Autodesk Inventor part; units mm, degrees
ref_plane "YZ Plane" through (0, 0, 0) normal (1, 0, 0) x (0, 1, 0)
ref_plane "XZ Plane" through (0, 0, 0) normal (0, 1, 0) x (-1, 0, 0)
ref_plane "XY Plane" through (0, 0, 0) normal (0, 0, 1) x (1, 0, 0)
sketch "Skizze1" plane through (0, 0, 0) normal (0, 0, 1) x (1, 0, 0)
  line L0 (-45, 15) -> (45, 15)
  line L1 (45, 15) -> (45, -15)
  line L2 (45, -15) -> (-45, -15)
  line L3 (-45, -15) -> (-45, 15)
  line L4 (-45, 15) -> (45, -15) construction
  line L5 (45, 15) -> (-45, -15) construction
  point P0 (0, 0)
  dimension "d0" = 30
  dimension "d1" = 90
extrude "Extrusion1" add sketch "Skizze1" along normal blind 1
sketch "Skizze4" plane through (0, 0, 1) normal (0, 0, 1) x (1, 0, 0)
  line L0 (15, -12.1) -> (-15, -12.1) construction
  line L1 (15, -11.2) -> (-15, -11.2)
  line L2 (-15, -13) -> (15, -13)
  arc A0 (15, -13) -> (15, -11.2) centre (15, -12.1) ccw
  arc A1 (-15, -11.2) -> (-15, -13) centre (-15, -12.1) ccw
  line L3 (0, 21) -> (0, -21)
  line L4 (-45, -15) -> (45, -15)
  point P0 (0, 0)
  point P1 (0, -12.1)
  dimension "d25" = 1.8
  dimension "d26" = 30
  dimension "d27" = 2
extrude "Extrusion2" cut sketch "Skizze4" against normal through all
sketch "Skizze2" plane through (0, 0, 1) normal (0, 0, 1) x (1, 0, 0)
  line L0 (31, 6) -> (-31, 6) construction
  line L1 (45, 15) -> (-45, 15)
  line L2 (0, 21) -> (0, -21)
  line L3 (-45, -15) -> (45, -15)
  dimension "d5" = 62
  dimension "d48" = 21
hole "Bohrung1" at (-31, 6, 1) at (31, 6, 1) direction (0, 0, -1) diameter 3.1 end through all
sketch "Skizze5" plane through (0, 0, 1) normal (0, 0, 1) x (1, 0, 0)
  line L0 (-45, -15) -> (45, -15)
  line L1 (0, 21) -> (0, -21)
  point P0 (0, 0)
  point P1 (22.05, -8.3)
  point P2 (-22.05, -8.3)
  dimension "d30" = 6.7
  dimension "d31" = 44.1
hole "Bohrung3" at (22.05, -8.3, 1) at (-22.05, -8.3, 1) direction (0, 0, -1) diameter 2.1 end through all
sketch "Skizze7" plane through (0, 0, 1) normal (0, 0, 1) x (1, 0, 0)
  line L0 (0, 21) -> (0, -21)
  line L1 (-45, -15) -> (45, -15)
  line L2 (-22, 15) -> (-14, 15)
  line L3 (-14, 15) -> (-14, 2)
  line L4 (-14, 2) -> (-22, 2)
  line L5 (-22, 2) -> (-22, 15)
  line L6 (-18, 2) -> (-18, 15) construction
  line L7 (45, 15) -> (-45, 15) construction
  point P0 (0, 0)
  dimension "d49" = 18
  dimension "d50" = 17
  dimension "d51" = 8
extrude "Extrusion4" cut sketch "Skizze7" against normal through all
chamfer "Fase1" distance 1 angle 45 2 edges at (-22, 2, 0.5) (-14, 2, 0.5)
properties part number "Ballsensorplatine" material "Phenolharz"
Could you check a few things on this model? Use its own coordinates, in mm. Coordinates: 2 decimals unless noted, no trailing zeros. Write each loop counter-clockwise with the first axis right and the second up, starting at its lowest first coordinate (ties: lowest second). Pieces come first, ordered by that corner, then holes. Notation, with made-up numbers: (-19.75, 41) -> (27.25, 41) arc R20 cw to (27.25, 76) -> close; hole circle Ø10 at (46.5, 41). An arc over 180 degrees is marked (long way). One line per question, with ' | ' between items. Start each with the question number.
1. If we section it at A-A (x = 12): Please give me the cut outline in (y, z), and give its area (3 significant figures).
2. If we section it at C-C (z = 0.3): Please give me the cut outline in (x, y), and give its area (3 significant figures).
3. Please list where these lines run through material, in increasing order: line 1 along X through (y, z) = (6, 0.5); line 2 along X through (y, z) = (-8.3, 0.5); line 3 along Y through (x, z) = (22.05, 0.35).
4. If we section it at D-D (x = -18): Please give me the cut outline in (y, z).
5. If we section it at B-B (y = -12.1): Please give me the cut outline in (x, z), and give its area (3 significant figures).
6. Thinking about a two-plate mould opening in Y: for faces 1 (the face through (-21.025, -8.072, 0.493)), 2 (the face through (29.463, 6.202, 0.493)), 3 (the face through (-1, 0, 0)), which applies, pulls with the +Y half, pulls with the -Y half, needs draft (parallel to the pull), parting line crosses it, or undercut?
7. Will these pins go through, and if not, where does the flat tip stop? P1, Ø0.5, axis at x = -16.5, z = 0.5, coming from the +Y side; P2, Ø5, axis at x = -31, y = 6, coming from the +Z side.
Return value:
1) outline: (-15, 0) -> (-13, 0) -> (-13, 1) -> (-15, 1) -> close; (-11.2, 0) -> (15, 0) -> (15, 1) -> (-11.2, 1) -> close | area: 28.2 mm²
2) outline: (-45, -15) -> (45, -15) -> (45, 15) -> (-14, 15) -> (-14, 3) -> (-15, 2) -> (-21, 2) -> (-22, 3) -> (-22, 15) -> (-45, 15) -> close; hole circle Ø3.1 at (-31, 6); hole circle Ø2.1 at (-22.05, -8.3); hole (-15, -13) -> (15, -13) arc R0.9 ccw to (15, -11.2) -> (-15, -11.2) arc R0.9 ccw to start; hole circle Ø2.1 at (22.05, -8.3); hole circle Ø3.1 at (31, 6) | area: 2,520 mm²
3) line 1: x = -45 to -32.55, -29.45 to -22, -14 to 29.45, 32.55 to 45 | line 2: x = -45 to -23.1, -21 to 21, 23.1 to 45 | line 3: y = -15 to -9.35, -7.25 to 15
4) outline: (-15, 0) -> (2, 0) -> (2, 1) -> (-15, 1) -> close
5) outline: (-45, 0) -> (-15.9, 0) -> (-15.9, 1) -> (-45, 1) -> close; (15.9, 0) -> (45, 0) -> (45, 1) -> (15.9, 1) -> close | area: 58.2 mm²
6) face 1: undercut | face 2: undercut | face 3: needs draft
7) P1: stops at y = 2 | P2: stops at z = 1
